Input: part model. Units: mm. Frame: model coordinates. A direction names the side the tool comes from. Round coordinates to 2 decimals unless told otherwise and drop trailing zeros. Loops run counter-clockwise (first coordinate to the right, second up) from the corner with the lowest first, then second, coordinate; pieces in that order, holes last. Notation, with made-up numbers: (35.25, 79) - (69.25, 79) arc R22 cw to (69.25, 112) - close; hole circle Ø1 at (65, -3.5). An arc over 180 degrees is marked (long way). Use CSV: the item, a comma, the result in double quotes. Start each with the question number.
1. Pin query (flat end, axial travel): P1, Ø7.5, axis at x = 6, y = -7, coming from the -Z side; P2, Ø3.5, axis at x = 5.49, y = -10, coming from the -Z side. Return the tip coordinate at first contact, or that it passes through.
2. Cut plane D-D (x = 10.25). Return loops of the section in (y, z).
3. Cut plane B-B (z = -4.25). Return loops of the section in (x, y), and give its area (3 significant figures).
4. Material intervals for probe 1 along X at (y, z) = (-16.25, -3.75); probe 2 along X at (y, z) = (-10, 4.05); probe 3 along Z at (x, y) = (2.75, -10), sorted ascending. Write a range as from..to.
5. Cut plane A-A (y = -10). Return loops of the section in (x, z).
6. Access query for faces 1 (the flat face through (12.91, -10, -1)), 2 (the cylindrical face through (4.75, -8.58, 3.17)), 3 (the flat face through (-2.09, -10, -5)). Directions: +Z, -Z, +X, -X, +Y, -Y. A direction counts if a zero-diameter tool reaches every point of the face in a straight line with its end or side. Return the directions, or none.
7. Cut plane C-C (y = -13.75). Return loops of the section in (x, z), and give its area (3 significant figures).
8. Pull-direction query (X, two-part tool) for faces 4 (the cylindrical face through (-1.5, -9.9, -2.7)), 5 (the flat face through (-3.59, -10, 0)), 6 (the flat face through (5, 0, 2)); classes: +X half, -X half, draft (parallel to the pull), parting line (faces both ways), or undercut.
```python
from build123d import *

# Parameters (mm, degrees)
F1_DEPTH       = 20
F3_D           = 3.2
F3_CSINK_D     = 5.5
F3_CSINK_ANGLE = 90
F4_DEPTH       = 20


with BuildPart() as f1:
    # F0 (on Front) → F1 (new body)
    with BuildSketch(Plane.XZ):
        with BuildLine():
            Line((14.4104288965, 5.1363992399), (-3.5895711035, 5.1363992399))
            Line((-3.5895711035, 5.1363992399), (-3.5895711035, 0.1363992399))
            Line((-3.5895711035, 0.1363992399), (-3.5895711035, -5.1626007601))
            ThreePointArc((-3.5895711035, -5.1626007601), (-3.1502312752, -6.2232609319), (-2.0895711035, -6.6626007601))
            Line((-2.0895711035, -6.6626007601), (-2.0895711035, -3.2634044741))
            Line((-2.0895711035, -3.2634044741), (-2.0895711035, -2.0636007601))
            Line((-2.0895711035, -2.0636007601), (-2.0895711035, 0.1363992399))
            Line((-2.0895711035, 0.1363992399), (5.4104288965, 0.1363992399))
            Line((5.4104288965, 0.1363992399), (12.9104288965, 0.1363992399))
            Line((12.9104288965, 0.1363992399), (12.9104288965, -2.0636007601))
            Line((12.9104288965, -2.0636007601), (12.9104288965, -3.2631007601))
            Line((12.9104288965, -3.2631007601), (12.9104288965, -6.6626007601))
            ThreePointArc((12.9104288965, -6.6626007601), (13.9710890683, -6.2232609319), (14.4104288965, -5.1626007601))
            Line((14.4104288965, -5.1626007601), (14.4104288965, -0.620780386))
            Line((14.4104288965, -0.620780386), (14.4104288965, 0.1363992399))
            Line((14.4104288965, 0.1363992399), (14.4104288965, 5.1363992399))
        make_face()
    extrude(amount=F1_DEPTH)

    # F3 (through all)
    with Locations(Plane(origin=(0, 0, 0), x_dir=(1, 0, 0), z_dir=(0, 0, -1))):
        with Locations((5.4901805706, 10)):
            CounterSinkHole(F3_D / 2, F3_CSINK_D / 2, counter_sink_angle=F3_CSINK_ANGLE)

    # F0 (on Front) → F4 (join)
    with BuildSketch(Plane.XZ):
        with BuildLine():
            Line((-2.0895711035, -2.0636007601), (-2.0895711035, -3.2634044741))
            ThreePointArc((-2.0895711035, -3.2634044741), (-1.5004229232, -2.6635026171), (-2.0895711035, -2.0636007601))
        make_face()
        with BuildLine():
            ThreePointArc((12.9104288965, -2.0636007601), (12.3277476003, -2.6633507601), (12.9104288965, -3.2631007601))
            Line((12.9104288965, -3.2631007601), (12.9104288965, -2.0636007601))
        make_face()
    extrude(amount=F4_DEPTH)


solid = f1.part
```
Established:
1,P1,"stops at z = 0.14"
1,P2,"stops at z = 1"
2,outline,"(-20, 0.14) - (0, 0.14) - (0, 5.14) - (-20, 5.14) - close"
3,outline,"(-3.59, -20) - (-2.09, -20) - (-2.09, 0) - (-3.59, 0) - close; (12.91, -20) - (14.41, -20) - (14.41, 0) - (12.91, 0) - close"
3,area,"60.0 mm2"
4,probe 1,"x = -3.59..-2.09, 12.91..14.41"
4,probe 2,"x = -3.59..3.89, 7.09..14.41"
4,probe 3,"z = 0.14..5.14"
5,outline,"(-3.59, -5.16) arc R1.5 ccw to (-2.09, -6.66) - (-2.09, -3.26) arc R0.6 ccw to (-2.09, -2.06) - (-2.09, 0.14) - (2.88, 0.14) - (3.89, 1.15) - (3.89, 5.14) - (-3.59, 5.14) - close; (7.09, 1.15) - (8.1, 0.14) - (12.91, 0.14) - (12.91, -2.06) arc R0.6 ccw to (12.91, -3.26) - (12.91, -6.66) arc R1.5 ccw to (14.41, -5.16) - (14.41, 5.14) - (7.09, 5.14) - close"
6,face 1,"+Y, -Y"
6,face 2,"+Z, -Z"
6,face 3,"-Z, +Y, -Y"
7,outline,"(-3.59, -5.16) arc R1.5 ccw to (-2.09, -6.66) - (-2.09, -3.26) arc R0.6 ccw to (-2.09, -2.06) - (-2.09, 0.14) - (12.91, 0.14) - (12.91, -2.06) arc R0.6 ccw to (12.91, -3.26) - (12.91, -6.66) arc R1.5 ccw to (14.41, -5.16) - (14.41, 5.14) - (-3.59, 5.14) - close"
7,area,"111 mm2"
8,face 4,"undercut"
8,face 5,"-X half"
8,face 6,"draft"
